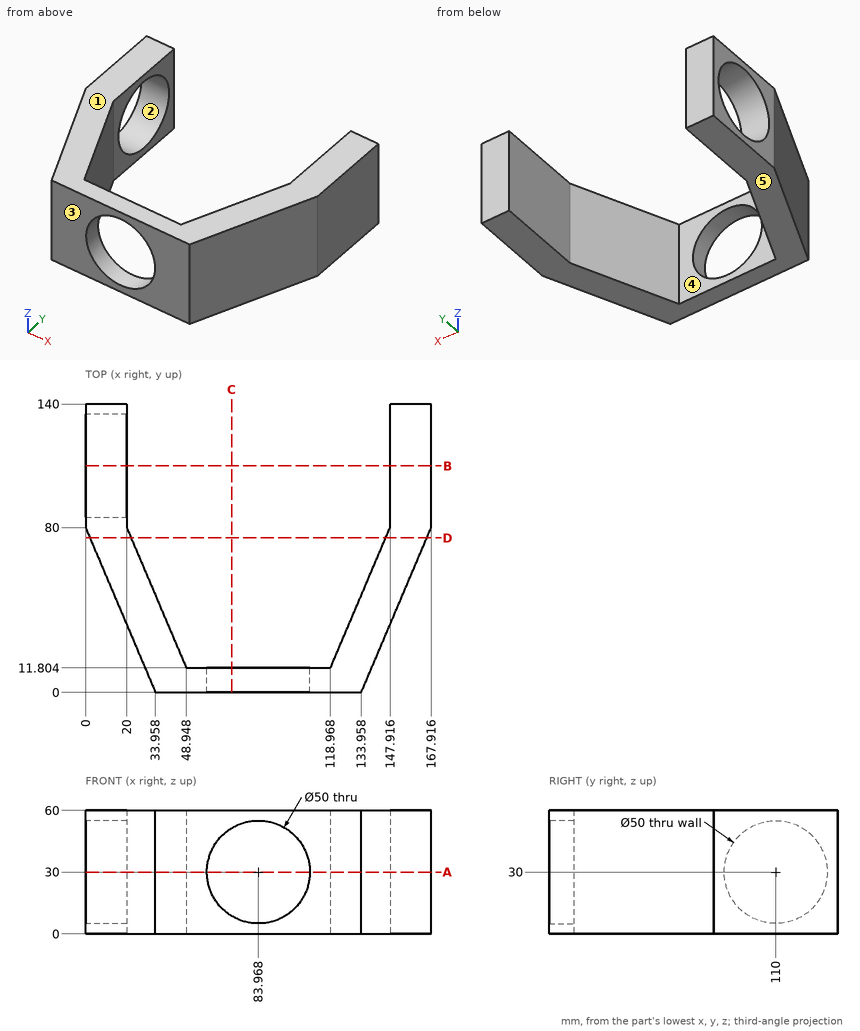
Geometry: see drawing. Coordinates: mm, zero at the bounding-box minimum. A direction names the side the tool comes from. Give positions to 0.01 mm unless a question says otherwise; leave off trailing zeros. Write each loop counter-clockwise with the first axis right and the second up, starting at its lowest first coordinate (ties: lowest second). Pieces come first, ordered by that corner, then holes. Notation, with made-up numbers: M -36.75,-35.75 L -27.75,-35.75 A23 ccw -27.75,-26.75 Z; hole C -17,-6.5 d6. An arc over 180 degrees is marked long. Answer as a JSON object with one key per item and string values.
Q1. Contact query for flat-ended pins moving along their axis: P1, Ø18, axis at x = 100.5, z = 39, coming from the +Y side; P2, Ø5, axis at y = 32, z = 33, coming from the -X side; P3, Ø3, axis at y = 58, z = 16.5, coming from the -X side. Output: stop coordinate, or through.
Geometry check:
{"P1": "stops at y = 11.8", "P2": "stops at x = 19.31", "P3": "stops at x = 8.7"}
Q2. Access query for the marked faces 4 and 5. Directions: +Z, -Z, +X, -X, +Y, -Y. A direction counts if a zero-diameter tool reaches every point of the face in a straight line with its end or side. Return the directions, or none.
Geometry check:
{"face 4": "+Z, -Z, +Y", "face 5": "-Z, +X, -X, +Y, -Y"}
Q3. Cut plane B-B, the plane y = 110. Return the cut outline in (x, z).
Geometry check:
{"outline": "M 0,0 L 20,0 L 20,5 L 0,5 Z; M 0,55 L 20,55 L 20,60 L 0,60 Z; M 147.92,0 L 167.92,0 L 167.92,60 L 147.92,60 Z"}
Q4. Ray query, line 1 along Z through (x, y) = (13, 110); line 2 along Y through (x, z) = (103, 51.5); line 3 along X through (y, z) = (55.5, 26) (1 decimal). Return the intervals inside material, ascending.
Geometry check:
{"line 1": "z = 0 to 5, 55 to 60", "line 2": "y = 0 to 11.8", "line 3": "x = 10.4 to 30.4, 137.5 to 157.5"}
Q5. Cut plane A-A, the plane z = 30. Return the cut outline in (x, y).
Geometry check:
{"outline": "M 0,80 L 33.96,0 L 58.97,0 L 58.97,11.8 L 48.95,11.8 L 20,80 L 20,85 L 0,85 Z; M 0,135 L 20,135 L 20,140 L 0,140 Z; M 108.97,0 L 133.96,0 L 167.92,80 L 167.92,140 L 147.92,140 L 147.92,80 L 118.97,11.8 L 108.97,11.8 Z"}
Q6. Cut plane D-D, the plane y = 75. Return the cut outline in (x, z).
Geometry check:
{"outline": "M 2.12,0 L 22.12,0 L 22.12,60 L 2.12,60 Z; M 145.79,0 L 165.79,0 L 165.79,60 L 145.79,60 Z"}
Q7. Mould query, pull axis Y, two halves, no side actions, for the marked faces 1, 2 and 3. Classes: +Y half, -Y half, draft (parallel to the pull), parting line (faces both ways), or undercut.
Geometry check:
{"face 1": "draft", "face 2": "undercut", "face 3": "-Y half"}
Q8. Cut plane C-C, the plane x = 71. Return the cut outline in (y, z).
Geometry check:
{"outline": "M 0,0 L 11.8,0 L 11.8,8.63 L 0,8.63 Z; M 0,51.37 L 11.8,51.37 L 11.8,60 L 0,60 Z"}
